Study the drawing (mm; zero at the part's minimum x, y, z) and answer. A direction names the side the tool comes from. Give positions to 0.01 mm unless a question says otherwise; leave off trailing zeros. Loops run counter-clockwise (first coordinate to the right, second up) from the corner with the lowest first, then second, coordinate; pieces in that order, holes last. Notation, with made-up numbers: M 21.5,58.25 L 42.5,58.25 A16 cw 42.5,64.25 Z; hole C -9.5,41.25 d5. An arc over 180 degrees is marked long. Return JSON: item names as keys, results as strings.
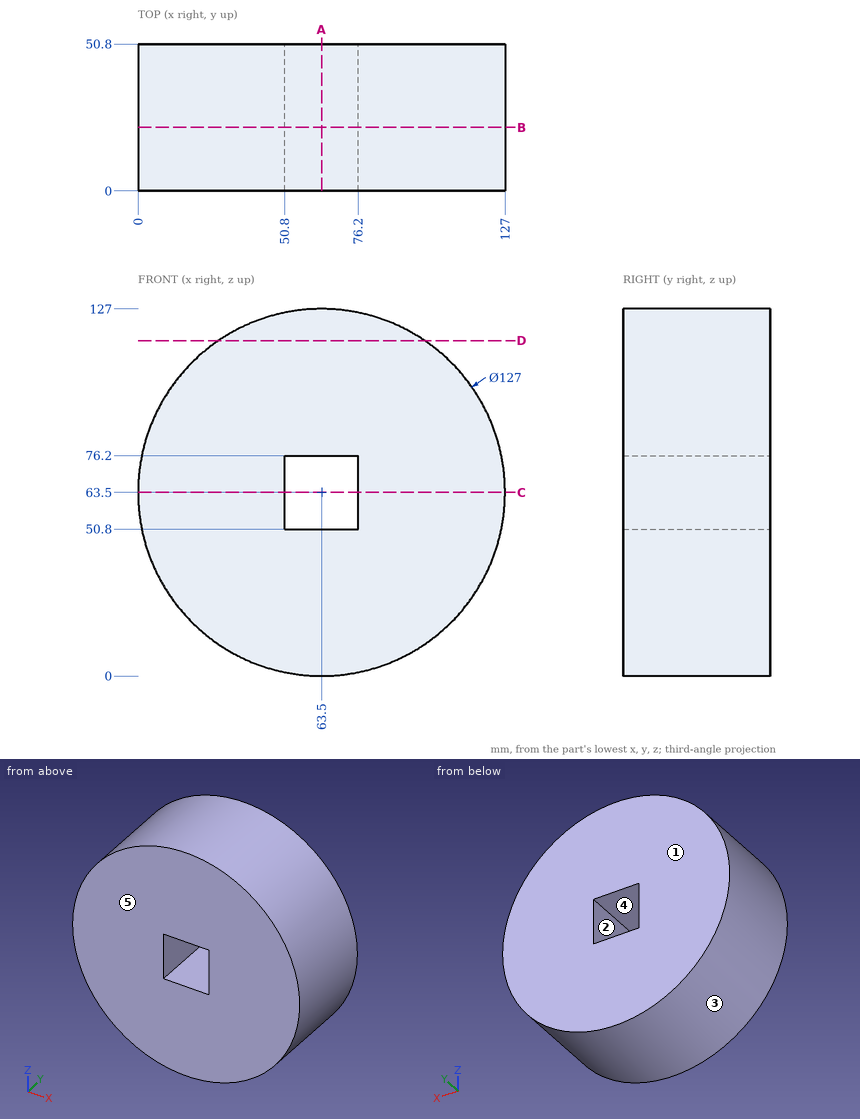
(1) Determine the mould class of the marked faces 3, 4 and 5 for opening direction X: released by +X, released by -X, zero draft, split by the parting line, or undercut.
Values follow:
{"face 3": "split by the parting line", "face 4": "undercut", "face 5": "zero draft"}
(2) The part is cut by section C-C (z = 63.5). Determine the outline of the cut face in (x, y), and give its area (3 significant figures).
Values follow:
{"outline": "M 0,0 L 50.8,0 L 50.8,50.8 L 0,50.8 Z; M 76.2,0 L 127,0 L 127,50.8 L 76.2,50.8 Z", "area": "5,160 mm²"}
(3) A tool of negligible diameter and unlimited length cuts with its end or side. For the marked faces 1 and 2, from which of +Z, -Z, +X, -X, +Y, -Y can it reach the whole face along a straight path? Write none if from no direction.
Values follow:
{"face 1": "+Z, -Z, +X, -X, +Y", "face 2": "+Y, -Y"}
(4) Straight lines are drawn through the part: line 1 along Z through (x, y) = (62.5, 3.5); line 2 along X through (y, z) = (25.5, 67.5); line 3 along Z through (x, y) = (90, 14). For each, find the intervals that lie inside material, in ascending order.
Values follow:
{"line 1": "0.01 to 50.8, 76.2 to 126.99", "line 2": "0.13 to 50.8, 76.2 to 126.87", "line 3": "5.79 to 121.21"}
(5) Given pin 1 (1 mm diameter, centred on y = 6.5, z = 77.5, fed in from +X); pin 2 (1.5 mm diameter, centred on x = 108.5, y = 11.5, fed in from -Z); pin 3 (8 mm diameter, centred on x = 53, y = 27, fed in from -Z), each flat-ended and moving along its own axis, determine where each tip first touches the part or whether it passes through.
Values follow:
{"pin 1": "x = 125.55", "pin 2": "z = 17.96", "pin 3": "z = 0.33"}
(6) The part is cut by section D-D (z = 116). Determine the outline of the cut face in (x, y), and give its area (3 significant figures).
Values follow:
{"outline": "M 27.78,0 L 99.22,0 L 99.22,50.8 L 27.78,50.8 Z", "area": "3,630 mm²"}
(7) The part is cut by section B-B (y = 22). Determine the outline of the cut face in (x, z).
Values follow:
{"outline": "C 63.5,63.5 d127; hole M 50.8,50.8 L 76.2,50.8 L 76.2,76.2 L 50.8,76.2 Z"}
(8) The part is cut by section A-A (x = 63.5). Determine the outline of the cut face in (y, z).
Values follow:
{"outline": "M 0,0 L 50.8,0 L 50.8,50.8 L 0,50.8 Z; M 0,76.2 L 50.8,76.2 L 50.8,127 L 0,127 Z"}
